Autodesk Inventor part; units mm, degrees
ref_plane "YZ Plane" through (0, 0, 0) normal (1, 0, 0) x (0, 1, 0)
ref_plane "XZ Plane" through (0, 0, 0) normal (0, 1, 0) x (-1, 0, 0)
ref_plane "XY Plane" through (0, 0, 0) normal (0, 0, 1) x (1, 0, 0)
sketch "Sketch1" plane through (0, 0, 0) normal (0, 0, 1) x (1, 0, 0)
  line L0 (0, 0) -> (25.4, 0)
  line L1 (25.4, 0) -> (25.4, 25.4)
  line L2 (25.4, 25.4) -> (0, 25.4)
  line L3 (0, 25.4) -> (0, 0)
  line L4 (3.175, 3.175) -> (22.225, 3.175)
  line L5 (22.225, 3.175) -> (22.225, 22.225)
  line L6 (22.225, 22.225) -> (3.175, 22.225)
  line L7 (3.175, 22.225) -> (3.175, 3.175)
  dimension "d0" = 25.4
  dimension "d1" = 25.4
  dimension "d2" = 19.05
  dimension "d3" = 19.05
  dimension "d4" = 3.175
  dimension "d5" = 3.175
extrude "Extrusion1" add sketch "Sketch1" along normal blind 587.375
sketch "Sketch2" plane through (0, 25.4, 0) normal (0, 1, 0) x (1, 0, 0)
  line L0 (25.4, 0) -> (0, 0)
  line L1 (0, 0) -> (0, -587.375)
  point P0 (12.7, -12.7)
  point P1 (12.7, -139.7)
  dimension "d8" = 12.7
  dimension "d9" = 12.7
  dimension "d10" = 12.7
  dimension "d11" = 139.7
hole "Hole1" at (12.7, 25.4, 12.7) at (12.7, 25.4, 139.7) direction (0, -1, 0) diameter 6.35 end through all
sketch "Sketch3" plane through (25.4, 0, 0) normal (1, 0, 0) x (0, 0, -1)
  line L0 (-587.375, 0) -> (-587.375, 25.4)
  line L1 (0, 0) -> (-587.375, 0)
  point P0 (-574.675, 12.7)
  point P1 (-549.275, 12.7)
  point P2 (-336.55, 12.7)
  point P3 (-311.15, 12.7)
  dimension "d19" = 12.7
  dimension "d20" = 12.7
  dimension "d21" = 12.7
  dimension "d22" = 25.4
  dimension "d23" = 212.725
  dimension "d24" = 25.4
  dimension "d25" = 12.7
  dimension "d26" = 12.7
hole "Hole2" at (25.4, 12.7, 574.675) at (25.4, 12.7, 549.275) at (25.4, 12.7, 336.55) at (25.4, 12.7, 311.15) direction (-1, 0, 0) diameter 6.35 end through all
sketch "Sketch6" plane through (0, 25.4, 0) normal (0, 1, 0) x (1, 0, 0)
  circle A0 centre (12.7, -12.7) radius 3.175
  circle A1 centre (12.7, -139.7) radius 3.175
  line L0 (25.4, 0) -> (0, 0)
  line L1 (0, 0) -> (0, -587.375)
  line L2 (25.4, -587.375) -> (0, -587.375)
  line L3 (25.4, 0) -> (25.4, -587.375)
  line L4 (25.4, -587.375) -> (3.175, -587.375)
  line L5 (0, -587.375) -> (25.4, -587.375)
  line L6 (25.4, -587.375) -> (25.4, -536.575)
  line L7 (25.4, 0) -> (25.4, -587.375)
  line L8 (25.4, -536.575) -> (3.175, -587.375)
  dimension "d41" = 22.225
  dimension "d42" = 50.8
extrude "Extrusion4" cut sketch "Sketch6" against normal blind 25.4 contours L3 L2 L8
sketch "Sketch7" plane through (0, 0, 0) normal (-1, 0, 0) x (0, 0, 1)
  line L0 (587.375, 25.4) -> (587.375, 0)
  line L1 (0, 25.4) -> (587.375, 25.4)
  point P0 (365.125, 12.7)
  point P1 (444.5, 12.7)
  point P2 (523.875, 12.7)
  dimension "d45" = 12.7
  dimension "d46" = 63.5
  dimension "d47" = 12.7
  dimension "d48" = 12.7
  dimension "d49" = 142.875
  dimension "d50" = 222.25
hole "Hole3" at (0, 12.7, 365.125) at (0, 12.7, 444.5) at (0, 12.7, 523.875) direction (1, 0, 0) diameter 6.35 end through all
properties part number "pickup arm 1x1" material "Aluminum 6061"
Verification items for the finished model (mm, model axes). A direction names the side the tool comes from. Round coordinates to 2 decimals unless told otherwise and drop trailing zeros. Loops run counter-clockwise (first coordinate to the right, second up) from the corner with the lowest first, then second, coordinate; pieces in that order, holes last. Notation, with made-up numbers: (-7, 84.25) - (45, 84.25) arc R25 cw to (45, 116.25) - close; hole circle Ø4 at (-27.75, 24). An arc over 180 degrees is marked (long way). Use a Markdown table: item, result. Add a question column.
1. Thickness scan on probe 1 along X at (y, z) = (1.7, 139.7) (3 decimals); probe 2 along X at (y, z) = (6, 104) (3 decimals). Record the ranges inside material, lowest first. Write a range as [from, to].
2. Access from +Z, -Z, +X, -X, +Y, -Y to the whole of each face (thin tool, end or side, straight path). Record for faces 1 (the face through (13, 0, 290)), 2 (the face through (3.175, 13, 290)).
3. Gauge pin test, flat ends, axial feed: pin 1 (7.5 mm diameter, centred on y = 12.7, z = 523.875, fed in from -X); pin 2 (7.5 mm diameter, centred on y = 12.7, z = 549.275, fed in from +X) (3 decimals). Record the tip position at first contact, or that the pin passes through.
4. Section check A-A, the plane z = 255. Record the boundary of the cut face in (x, y) (3 decimals).
5. Release check for a two-part mould opening along X. For faces 3 (the face through (17.632, 2.411, 554.331)), 4 (the face through (13, 25.4, 290)), 5 (the face through (22.225, 13, 268)) record: released by +X, released by -X, zero draft, split by the parting line, or undercut.
Checks:
| question | item | result |
|---|---|---|
| 1 | probe 1 | x = [0, 9.525], [15.875, 25.4] |
| 1 | probe 2 | x = [0, 3.175], [22.225, 25.4] |
| 2 | face 1 | +Z, -Z, +X, -X, -Y |
| 2 | face 2 | +Z, -Z |
| 3 | pin 1 | stops at x = 0 |
| 3 | pin 2 | stops at x = 3.175 |
| 4 | outline | (0, 0) - (25.4, 0) - (25.4, 25.4) - (0, 25.4) - close; hole (3.175, 3.175) - (22.225, 3.175) - (22.225, 22.225) - (3.175, 22.225) - close |
| 5 | face 3 | released by +X |
| 5 | face 4 | zero draft |
| 5 | face 5 | undercut |
